For this review, take the finished solid that the model builds, in its own axes (mm). A direction names the side the tool comes from. Round coordinates to 2 decimals unless told otherwise and drop trailing zeros. Loops run counter-clockwise (first coordinate to the right, second up) from the corner with the lowest first, then second, coordinate; pieces in that order, holes last. Notation, with made-up numbers: (-10, 36.5) -> (17, 36.5) arc R23 cw to (17, 53.5) -> close; hole circle Ø11 at (-37.75, -10). An arc over 180 degrees is marked (long way). Write each question's results on one line, items separated by ' | '.
```python
from build123d import *

# Parameters (mm, degrees)
BOSS_EXTRUDE1_DEPTH                  = 25.4
F_15_64_0_23438_DIAMETER_HOLE1_D     = 5.953252
F_15_64_0_23438_DIAMETER_HOLE1_DEPTH = 25.4
F_15_64_0_23438_DIAMETER_HOLE1_TIP   = 1.788537341
F_1_4_CLEARANCE_HOLE1_D              = 6.7564
F_1_4_CLEARANCE_HOLE1_DEPTH          = 25.4
F_1_4_CLEARANCE_HOLE1_TIP            = 2.029827343
FILLET1_R                            = 2.54


with BuildPart() as part:
    # Sketch1 → Boss-Extrude1 (new body)
    with BuildSketch(Plane(origin=(0, 0, 0), x_dir=(0, 0, -1), z_dir=(1, 0, 0))):
        with BuildLine():
            Line((0, 0), (0, 25.908))
            Line((0, 25.908), (-5.08, 25.908))
            Line((-5.08, 25.908), (-5.08, 10.795))
            Line((-5.08, 10.795), (-13.97, 10.795))
            ThreePointArc((-13.97, 10.795), (-21.154204897, 7.819204897), (-24.13, 0.635))
            Line((-24.13, 0.635), (-24.13, -0.635))
            ThreePointArc((-24.13, -0.635), (-21.154204897, -7.819204897), (-13.97, -10.795))
            Line((-13.97, -10.795), (-5.08, -10.795))
            Line((-5.08, -10.795), (-5.08, -25.908))
            Line((-5.08, -25.908), (0, -25.908))
            Line((0, -25.908), (0, 0))
        make_face()
    extrude(amount=-BOSS_EXTRUDE1_DEPTH)

    # 15/64 (0.23438) Diameter Hole1
    with Locations(Plane(origin=(0, 0, 0), x_dir=(0, 0, -1), z_dir=(1, 0, 0))):
        with Locations((-14.2875, 0)):
            Hole(F_15_64_0_23438_DIAMETER_HOLE1_D / 2, depth=F_15_64_0_23438_DIAMETER_HOLE1_DEPTH)
            with Locations((0, 0, -(F_15_64_0_23438_DIAMETER_HOLE1_DEPTH + F_15_64_0_23438_DIAMETER_HOLE1_TIP / 2))):  # 118° drill point
                Cone(0, F_15_64_0_23438_DIAMETER_HOLE1_D / 2, F_15_64_0_23438_DIAMETER_HOLE1_TIP, mode=Mode.SUBTRACT)

    # 1/4 Clearance Hole1
    with Locations(Plane.XY.offset(5.08)):
        with Locations((-12.7, 19.558), (-12.7, -19.558)):
            Hole(F_1_4_CLEARANCE_HOLE1_D / 2, depth=F_1_4_CLEARANCE_HOLE1_DEPTH)
            with Locations((0, 0, -(F_1_4_CLEARANCE_HOLE1_DEPTH + F_1_4_CLEARANCE_HOLE1_TIP / 2))):  # 118° drill point
                Cone(0, F_1_4_CLEARANCE_HOLE1_D / 2, F_1_4_CLEARANCE_HOLE1_TIP, mode=Mode.SUBTRACT)

    # Fillet1
    fillet1_edges = [part.edges().sort_by_distance(p)[0] for p in [
        (0, -10.795, 9.525),
        (-25.4, -10.795, 9.525),
        (0, -7.819204897, 21.154204897),
        (-25.4, -7.819204897, 21.154204897),
        (0, -18.3515, 5.08),
        (-12.7, -25.908, 5.08),
        (0, 0, 24.13),
        (0, -25.908, 2.54),
        (0, 7.819204897, 21.154204897),
        (0, 0, 0),
        (0, 10.795, 9.525),
        (0, 25.908, 2.54),
        (0, 18.3515, 5.08),
        (-25.4, -25.908, 2.54),
        (-25.4, 0, 0),
        (-25.4, 25.908, 2.54),
        (-25.4, 18.3515, 5.08),
        (-25.4, 10.795, 9.525),
        (-25.4, 7.819204897, 21.154204897),
        (-25.4, 0, 24.13),
        (-12.7, -25.908, 0),
        (-12.7, 25.908, 0),
        (-12.7, 25.908, 5.08),
    ]]
    fillet(fillet1_edges, radius=FILLET1_R - 0.0001)  # a hair under: the kernel refuses the full size


solid = part.part
```
1. Consider section B-B (z = 12.25). State the section outline as (x, y) points (3 decimals).
Values found:
outline: (-25.4, -8.255) arc R2.54 ccw to (-22.86, -10.795) -> (-2.54, -10.795) arc R2.54 ccw to (0, -8.255) -> (0, -2.17) -> (-25.4, -2.17) -> close; (-25.4, 2.17) -> (0, 2.17) -> (0, 8.255) arc R2.54 ccw to (-2.54, 10.795) -> (-22.86, 10.795) arc R2.54 ccw to (-25.4, 8.255) -> close
2. Tool access review of faces 4 (the face through (-24.636, 15.706, 4.356)), 5 (the face through (-0.724, 10.031, 9.605)), 6 (the face through (-13, -10.795, 10)), 7 (the face through (-0.724, -15.917, 4.316)): name each direction out of +Z, -Z, +X, -X, +Y, -Y from which nothing blocks a thin tool from reaching the whole face with its end or side.
Values found:
face 4: +Z, -X, +Y | face 5: +Z, +X, +Y | face 6: +Z, +X, -X, -Y | face 7: +Z, +X, -Y
3. Consider section D-D (y = 0). State the section outline as (x, z) points, plus the area to 3 significant figures.
Values found:
outline: (-25.4, 2.54) arc R2.54 ccw to (-22.86, 0) -> (-2.54, 0) arc R2.54 ccw to (0, 2.54) -> (0, 11.31) -> (-25.4, 11.31) -> close; (-25.4, 17.26) -> (0, 17.26) -> (0, 21.59) arc R2.54 ccw to (-2.54, 24.13) -> (-22.86, 24.13) arc R2.54 ccw to (-25.4, 21.59) -> close | area: 456 mm2
4. Draft analysis for pull direction Z (two halves, no side actions). For faces 1 (the face through (-12.84, -25.14, 0.72)), 2 (the face through (-12.878, -1.14, 17.037)), 3 (the face through (-14.1, -25.2, 4.3)), state which applies: released by +Z, released by -Z, zero draft, split by the parting line, or undercut.
Values found:
face 1: released by -Z | face 2: undercut | face 3: released by +Z
5. To check wall thickness, follow probe 1 along Y at (x, z) = (-12.7, 3.05); probe 2 along Z at (x, y) = (-19.5, 0); probe 3 along Y at (x, z) = (-11.5, 1.25). State the ranges of each line that lie inside material, in increasing order.
Values found:
probe 1: y = -25.86 to -22.94, -16.18 to 16.18, 22.94 to 25.86 | probe 2: z = 0 to 11.31, 17.26 to 24.13 | probe 3: y = -25.56 to -22.72, -16.4 to 16.4, 22.72 to 25.56
6. For pin 1 (10 mm diameter, centred on x = -8, y = 19.5, fed in from +Z); pin 2 (2 mm diameter, centred on x = -18, z = 13.5, fed in from +Y) (3 decimals); pin 3 (6 mm diameter, centred on x = -9.5, y = 9, fed in from +Z); pin 4 (6 mm diameter, centred on y = 16, z = 14.5, fed in from -X), all flat-tipped, find the tip position at first contact; note any pin that passes through.
Values found:
pin 1: stops at z = 5.08 | pin 2: stops at y = 10.795 | pin 3: stops at z = 22.6 | pin 4: passes through
7. Consider section A-A (x = -12.7). Give the number of separate pieces and of enclosed holes in the cut face, plus the area to 3 significant figures.
Values found:
separate pieces: 3 | enclosed holes: 1 | area: 528 mm2
